```python
from build123d import *

# Parameters (mm, degrees)
SKETCH1_W           = 33.333333333
SKETCH1_H           = 33.333333333
SKETCH1_W_2         = 30.133333333
SKETCH1_H_2         = 30.133333333
BOSS_EXTRUDE1_DEPTH = 80
FILLET2_R           = 3
SCALE1_SCALE        = 7.5


with BuildPart() as part:
    # Sketch1 → Boss-Extrude1 (new body)
    with BuildSketch(Plane(origin=(0, 0, 0), x_dir=(1, 0, 0), z_dir=(0, 1, 0))):
        with Locations((16.666666666, 16.666666666)):
            Rectangle(SKETCH1_W, SKETCH1_H)
        with Locations((16.666666666, 16.666666666)):
            Rectangle(SKETCH1_W_2, SKETCH1_H_2, mode=Mode.SUBTRACT)
    extrude(amount=BOSS_EXTRUDE1_DEPTH)

    # Fillet2
    fillet2_edges = [part.edges().sort_by_distance(p)[0] for p in [
        (0, 40, -33.333333333),
        (33.333333333, 40, -33.333333333),
        (33.333333333, 40, 0),
        (0, 40, 0),
    ]]
    fillet(fillet2_edges, radius=FILLET2_R)


with BuildPart() as part_1:
    # Scale1: scaled about (16.666666667, 40, -16.666666667)
    add(part.part.scale(SCALE1_SCALE).moved(Location((-108.333333336, -260, 108.333333336))))


solid = part_1.part
```
Could you check a few things on this model? Use its own coordinates, in mm. A direction names the side the tool comes from. Coordinates: 2 decimals unless noted, no trailing zeros. Write each loop counter-clockwise with the first axis right and the second up, starting at its lowest first coordinate (ties: lowest second). Pieces come first, ordered by that corner, then holes. Notation, with made-up numbers: (7.25, 17.5) -> (16.25, 17.5) arc R22 ccw to (16.25, 38.5) -> close; hole circle Ø11 at (56, 46.5). An arc over 180 degrees is marked (long way). Return JSON: item names as keys, results as strings.
(1) Imagine slicing it at C-C, the plane y = -59.5. Please give me the cut outline in (x, z).
Numbers:
{"outline": "(-108.33, -119.17) arc R22.5 ccw to (-85.83, -141.67) -> (119.17, -141.67) arc R22.5 ccw to (141.67, -119.17) -> (141.67, 85.83) arc R22.5 ccw to (119.17, 108.33) -> (-85.83, 108.33) arc R22.5 ccw to (-108.33, 85.83) -> close; hole (-96.33, -129.67) -> (129.67, -129.67) -> (129.67, 96.33) -> (-96.33, 96.33) -> close"}
(2) Which directions (+Z, -Z, +X, -X, +Y, -Y) give clear straight access to the entire face, cutting with the end or side of a thin tool? Please do faces 4 (the flat face through (-96.333, 36, -15)), 5 (the cylindrical face through (-101.92, 44.2, -134.9)).
Numbers:
{"face 4": "+Y, -Y", "face 5": "-Z, -X, +Y, -Y"}
(3) I need wall thicknesses on L1, parallel to Z at x = -32, y = -109.5; L2, parallel to X at y = -172, z = -33; L3, parallel to X at y = 145, z = -123.5. Which ranges of each line are inside material? Lowest first, please.
Numbers:
{"L1": "z = -141.67 to -129.67, 96.33 to 108.33", "L2": "x = -108.33 to -96.33, 129.67 to 141.67", "L3": "x = -107.91 to -96.33, 129.67 to 141.25"}
(4) We'd pull the mould along X, two halves only. Please class faces 1 (the flat face through (16, 340, -138)), 2 (the cylindrical face through (-101.917, 44.2, 101.567)), 3 (the flat face through (15, 36, 96.333)): +X half, -X half, draft (parallel to the pull), parting line (faces both ways), or undercut.
Numbers:
{"face 1": "draft", "face 2": "-X half", "face 3": "undercut"}
(5) Imagine slicing it at A-A, the plane z = 52. Please give me the cut outline in (x, y).
Numbers:
{"outline": "(-108.33, -260) -> (-96.33, -260) -> (-96.33, 340) -> (-108.33, 340) -> close; (129.67, -260) -> (141.67, -260) -> (141.67, 340) -> (129.67, 340) -> close"}
(6) Imagine slicing it at B-B, the plane x = 75.5. Please give me the cut outline in (y, z), then the cut area to 3 significant figures.
Numbers:
{"outline": "(-260, -141.67) -> (340, -141.67) -> (340, -129.67) -> (-260, -129.67) -> close; (-260, 96.33) -> (340, 96.33) -> (340, 108.33) -> (-260, 108.33) -> close", "area": "14,400 mm2"}
